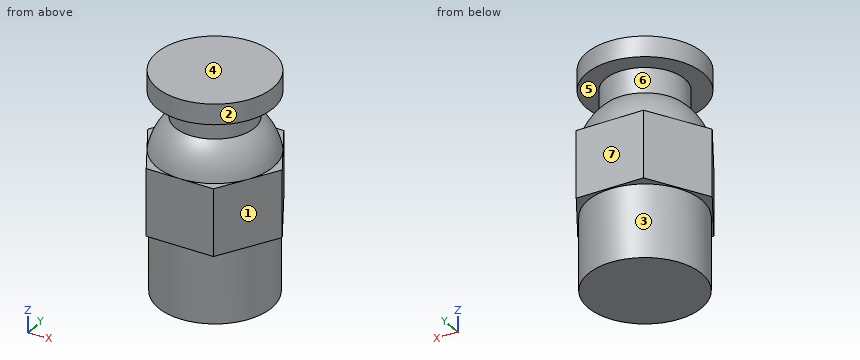
from build123d import *

# Parameters (mm, degrees)
SKETCH1_R           = 4.875
BOSS_EXTRUDE1_DEPTH = 6.25
BOSS_EXTRUDE2_DEPTH = 5.75
SKETCH3_R           = 5
BOSS_EXTRUDE3_DEPTH = 6.75


with BuildPart() as part:
    # Sketch1 → Boss-Extrude1 (new body)
    with BuildSketch(Plane.XY):
        Circle(SKETCH1_R)
    extrude(amount=BOSS_EXTRUDE1_DEPTH)

    # Sketch2 → Boss-Extrude2 (add)
    with BuildSketch(Plane.XY.offset(6.25)):
        Polygon((5.773502692, 0), (2.886751346, 5), (-2.886751346, 5), (-5.773502692, 0), (-2.886751346, -5), (2.886751346, -5), align=None)
    extrude(amount=BOSS_EXTRUDE2_DEPTH)

    # Sketch3 → Boss-Extrude3 (add)
    with BuildSketch(Plane.XY.offset(12)):
        with Locations(Location((0, 0, 0), (0, 0, 150))):
            Circle(SKETCH3_R)
    extrude(amount=BOSS_EXTRUDE3_DEPTH)

    # Sketch4 → Cut-Revolve1 (revolve, cut)
    with BuildSketch(Plane(origin=(0, 0, 0), x_dir=(0, 0, -1), z_dir=(1, 0, 0))):
        with BuildLine():
            Line((-17, 5), (-17, 3.4))
            Line((-17, 3.4), (-14.850952939, 3.4))
            ThreePointArc((-14.850952939, 3.4), (-13.557536702, 4.435310943), (-12, 5))
            Line((-12, 5), (-17, 5))
        make_face()
    revolve(axis=Axis((0, 0, 12), (0, 0, 1)), mode=Mode.SUBTRACT)


solid = part.part
Can you work these out from the model? Positions are in its coordinate system, mm. Face numbers are marked on the shaded views. A direction names the side the tool comes from. Coordinates: 2 decimals unless noted, no trailing zeros. Loops run counter-clockwise (first coordinate to the right, second up) from the corner with the lowest first, then second, coordinate; pieces in that order, holes last. Notation, with made-up numbers: M 15,50 L 38,50 A33 cw 38,80 Z; hole C 2.5,7 d2. An arc over 180 degrees is marked long. Return JSON: item names as keys, results as strings. Group by question number.
Item 1: If I drill on L1, parallel to Z at x = -2, y = 3.75; L2, parallel to Y at x = 4.5, z = 8.75; L3, parallel to Y at x = -2.5, z = 3, over which ranges is the centre line in solid material (lowest first)? Write a range as from..to.
Item 2: Imagine slicing it at C-C (z = 11.5). Please give me the cut outline in (x, y), and give its area (3 significant figures).
Item 3: I'm going to push a flat-ended pin straight in: pin 1 Ø1 at (x, y) = (3, 1.5) entering from -Z. Where does the tip first touch, or does it pass through?
Item 4: Thinking about a two-plate mould opening in Z: for the marked faces 4, 5, 6 and 7, which applies, released by +Z, released by -Z, zero draft, split by the parting line, or undercut?
Item 5: Imagine slicing it at D-D (x = -2.25). Please give me the cut outline in (y, z).
Item 6: Imagine slicing it at A-A (y = -4). Please give me the cut outline in (x, z).
Item 7: On a 3-axis mill with a long thin cutter (end or side, diameter ignored), from which of +Z, -Z, +X, -X, +Y, -Y can I reach the whole of each face in a straight line? I mean the marked faces 1, 2 and 3. Say none if no direction works.
Item 8: Imagine slicing it at B-B (y = 0.5). Please give me the cut outline in (x, z).
Verdict:
{
 "1": {"L1": "z = 0..13.86, 17..18.75", "L2": "y = -2.21..2.21", "L3": "y = -4.19..4.19"},
 "2": {"outline": "M -5.77,0 L -2.89,-5 L 2.89,-5 L 5.77,0 L 2.89,5 L -2.89,5 Z", "area": "86.6 mm^2"},
 "3": {"pin 1": "stops at z = 0"},
 "4": {"face 4": "released by +Z", "face 5": "undercut", "face 6": "undercut", "face 7": "zero draft"},
 "5": {"outline": "M -5,6.25 L -4.32,6.25 L -4.32,0 L 4.32,0 L 4.32,6.25 L 5,6.25 L 5,12 L 4.47,12 A4.56 ccw 2.55,14.85 L 2.55,17 L 4.47,17 L 4.47,18.75 L -4.47,18.75 L -4.47,17 L -2.55,17 L -2.55,14.85 A4.56 ccw -4.47,12 L -5,12 Z"},
 "6": {"outline": "M -3.46,6.25 L -2.79,6.25 L -2.79,0 L 2.79,0 L 2.79,6.25 L 3.46,6.25 L 3.46,12 L 3,12 A3.14 ccw -3,12 L -3.46,12 Z; M -3,17 L 3,17 L 3,18.75 L -3,18.75 Z"},
 "7": {"face 1": "+Z, -Z, +X, -Y", "face 2": "+Z", "face 3": "-Z"},
 "8": {"outline": "M -5.48,6.25 L -4.85,6.25 L -4.85,0 L 4.85,0 L 4.85,6.25 L 5.48,6.25 L 5.48,12 L 4.97,12 A5.06 ccw 3.36,14.85 L 3.36,17 L 4.97,17 L 4.97,18.75 L -4.97,18.75 L -4.97,17 L -3.36,17 L -3.36,14.85 A5.06 ccw -4.97,12 L -5.48,12 Z"}
}
